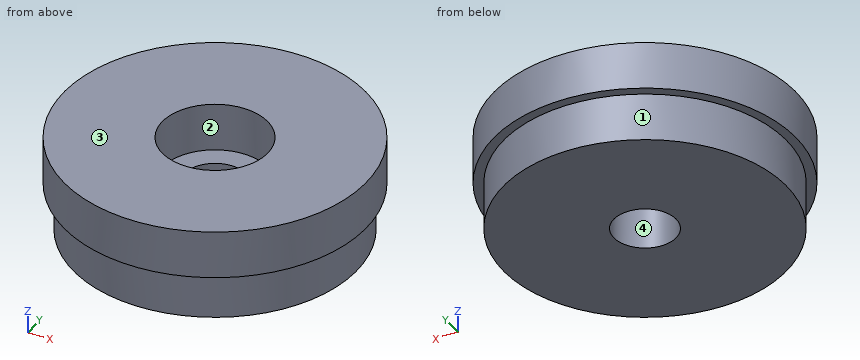
```python
from build123d import *

# Parameters (mm, degrees)
SKETCH1_R           = 8
SKETCH1_R_2         = 2.794
BOSS_EXTRUDE1_DEPTH = 2.54
SKETCH2_R           = 7.5
SKETCH2_R_2         = 1.651
BOSS_EXTRUDE2_DEPTH = 2.54


with BuildPart() as part:
    # Sketch1 → Boss-Extrude1 (new body)
    with BuildSketch(Plane.XY):
        Circle(SKETCH1_R)
        Circle(SKETCH1_R_2, mode=Mode.SUBTRACT)
    extrude(amount=-BOSS_EXTRUDE1_DEPTH)

    # Sketch2 → Boss-Extrude2 (add)
    with BuildSketch(Plane(origin=(0, 0, -2.54), x_dir=(-1, 0, 0), z_dir=(0, 0, -1))):
        Circle(SKETCH2_R)
        Circle(SKETCH2_R_2, mode=Mode.SUBTRACT)
    extrude(amount=BOSS_EXTRUDE2_DEPTH)


solid = part.part
```
CAD build for the part. Positions are in the model's coordinates, mm. Face numbers are marked on the shaded views. Round coordinates to 2 decimals unless told otherwise and drop trailing zeros. Order: outer loops, then holes, each group sorted by start corner. A loop starts at its lowest first (then second) coordinate and runs counter-clockwise, first axis right, second up. Notation, with made-up numbers: (1.5, 16.5) - (45.5, 16.5) arc R18 cw to (45.5, 28.5) - close; hole circle Ø7 at (-14, 48.5). An arc over 180 degrees is marked (long way). Answer in a Markdown table with one row per item. Add a question column.
(1) Mould opens along Y. For the marked faces 1, 2, 3 and 4 say: +Y half, -Y half, draft (parallel to the pull), parting line (faces both ways), or undercut.
(2) Band-saw the part on D-D on y = -4.75. List the corners of the cut face in (x, z), and give its area (3 significant figures).
(3) Probe L1, parallel to Y at x = 0, z = -3.5; L2, parallel to Y at x = 0, z = -1.5; L3, parallel to X at y = -2.5, z = -1.6. List the from-to ranges inside material, lowest first. Write a range as [from, to].
(4) Band-saw the part on C-C on z = -3.5. List the corners of the cut face in (x, y), and give its area (3 significant figures).
(5) Drop flat-ended pins along their axis: pin 1 Ø2 at (x, z) = (4.5, -3) entering from -Y; pin 2 Ø2 at (y, z) = (5, -2.5) entering from -X; pin 3 Ø1.7 at (x, y) = (0.5, 1.5) entering from +Z. Give the stop position or say it passes through.
(6) Band-saw the part on A-A on y = 0. List the corners of the cut face in (x, z).
Data:
| question | item | result |
|---|---|---|
| 1 | face 1 | parting line |
| 1 | face 2 | undercut |
| 1 | face 3 | draft |
| 1 | face 4 | undercut |
| 2 | outline | (-6.44, -2.54) - (-5.8, -2.54) - (-5.8, -5.08) - (5.8, -5.08) - (5.8, -2.54) - (6.44, -2.54) - (6.44, 0) - (-6.44, 0) - close |
| 2 | area | 62.2 mm^2 |
| 3 | L1 | y = [-7.5, -1.65], [1.65, 7.5] |
| 3 | L2 | y = [-8, -2.79], [2.79, 8] |
| 3 | L3 | x = [-7.6, -1.25], [1.25, 7.6] |
| 4 | outline | circle Ø15 at (0, 0); hole circle Ø3.3 at (0, 0) |
| 4 | area | 168 mm^2 |
| 5 | pin 1 | stops at y = -7.14 |
| 5 | pin 2 | stops at x = -6.93 |
| 5 | pin 3 | stops at z = -2.54 |
| 6 | outline | (-8, -2.54) - (-7.5, -2.54) - (-7.5, -5.08) - (-1.65, -5.08) - (-1.65, -2.54) - (-2.79, -2.54) - (-2.79, 0) - (-8, 0) - close; (1.65, -5.08) - (7.5, -5.08) - (7.5, -2.54) - (8, -2.54) - (8, 0) - (2.79, 0) - (2.79, -2.54) - (1.65, -2.54) - close |
